Input: dimensioned drawing with shaded views. Units: mm. Origin: part minimum x, y, z. A direction names the side the tool comes from. Coordinates: 2 decimals unless noted, no trailing zeros. Loops run counter-clockwise (first coordinate to the right, second up) from the corner with the lowest first, then second, coordinate; pieces in that order, holes last.
Item 1: Reachability of the marked faces 4 and 5 from +Z, -Z, +X, -X, +Y, -Y: full face, straight path, thin tool, end or side. Return the list, or none.
Item 2: Section C-C on y = 17.5. Return loops of the section in (x, z), and give its area (4 significant figures).
Item 3: Section A-A on z = 2.5. Return loops of the section in (x, y), and give its area (3 significant figures).
Item 4: Section B-B on x = 19.5. Return loops of the section in (y, z), and give its area (3 significant figures).
Item 5: Contact query for flat-ended pins moving along their axis: P1, Ø1.5, axis at x = 20, y = 20.5, coming from the -Z side; P2, Ø2, axis at x = 9.85, y = 23.5, coming from the -Z side; P3, Ø9.5, axis at x = 13.5, y = 14, coming from the +Z side; P4, Ø1.5, axis at x = 24.85, y = 3.5, coming from the -Z side. Output: stop coordinate, or through.
Item 6: Pull-direction query (Y, two-part tool) for the marked faces 1, 2 and 3; classes: released by +Y, released by -Y, zero draft, split by the parting line, or undercut.
Item 7: Ray query, line 1 along Y through (x, z) = (24.85, 6.5); line 2 along X through (y, z) = (3.5, 3); line 3 along Y through (x, z) = (24.85, 4.75). Return the intervals inside material, ascending.
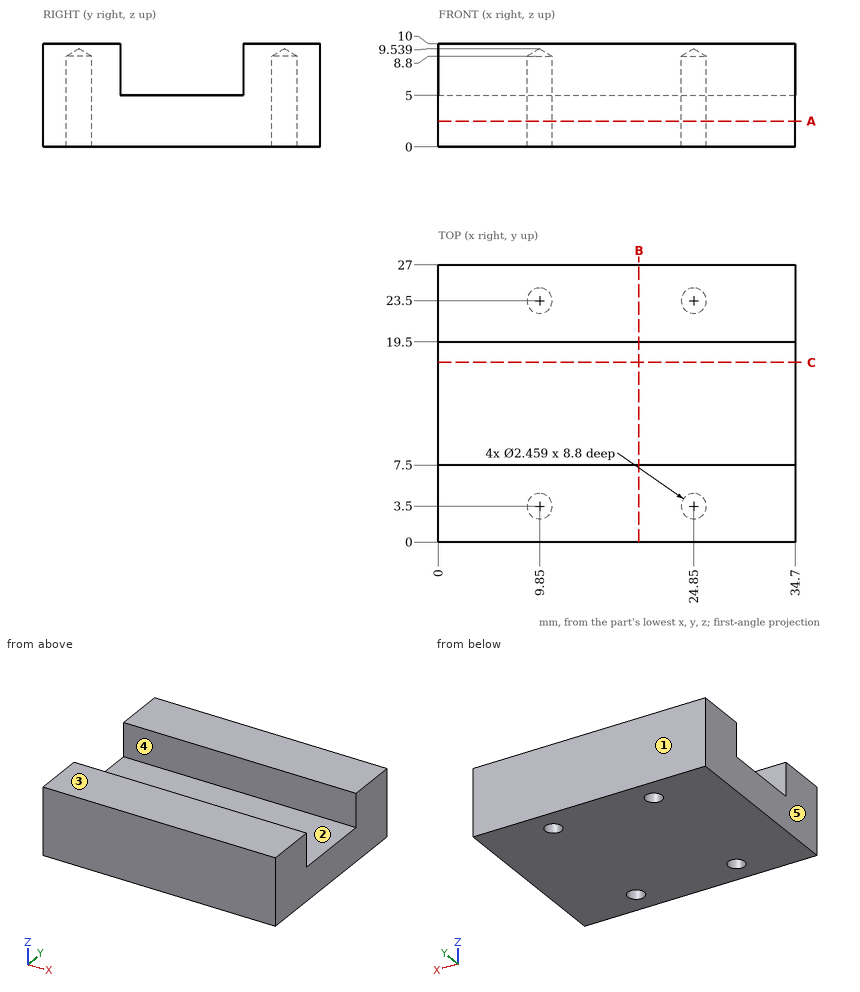
Results found:
1. face 4: +Z, +X, -X
1. face 5: +Z, -Z, -X, +Y, -Y
2. outline: (0, 0) - (34.7, 0) - (34.7, 5) - (0, 5) - close
2. area: 173.5 mm2
3. outline: (0, 0) - (34.7, 0) - (34.7, 27) - (0, 27) - close; hole circle Ø2.46 at (9.85, 3.5); hole circle Ø2.46 at (9.85, 23.5); hole circle Ø2.46 at (24.85, 3.5); hole circle Ø2.46 at (24.85, 23.5)
3. area: 918 mm2
4. outline: (0, 0) - (27, 0) - (27, 10) - (19.5, 10) - (19.5, 5) - (7.5, 5) - (7.5, 10) - (0, 10) - close
4. area: 210 mm2
5. P1: stops at z = 0
5. P2: stops at z = 8.94
5. P3: stops at z = 5
5. P4: stops at z = 9.09
6. face 1: released by +Y
6. face 2: undercut
6. face 3: zero draft
7. line 1: y = 0 to 2.27, 4.73 to 7.5, 19.5 to 22.27, 24.73 to 27
7. line 2: x = 0 to 8.62, 11.08 to 23.62, 26.08 to 34.7
7. line 3: y = 0 to 2.27, 4.73 to 22.27, 24.73 to 27
